Verification items for this drawing (mm, ordinates from the low corner). Coordinates: 2 decimals unless noted, no trailing zeros. Order: outer loops, then holes, each group sorted by start corner. A loop starts at its lowest first (then second) coordinate and runs counter-clockwise, first axis right, second up.
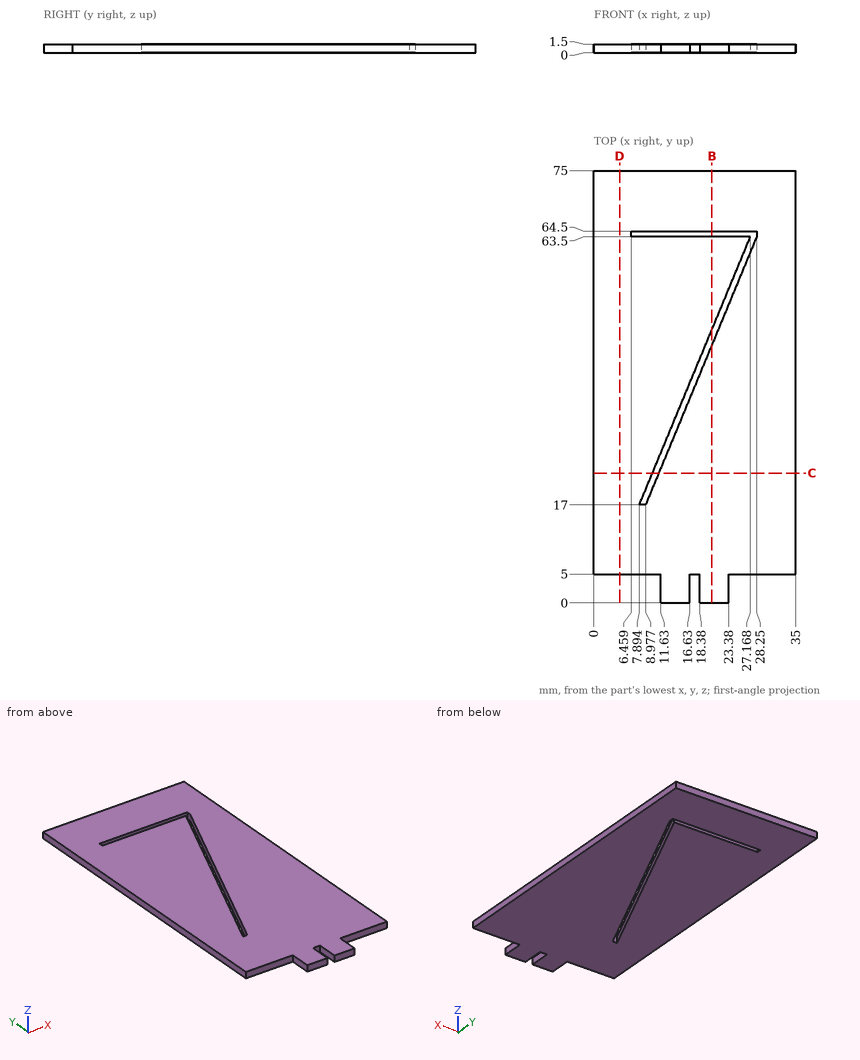
(1) Cross-section at B-B (x = 20.5). Enter the section's corners in (y, z), and give its area (3 significant figures).
Filled in:
outline: (0, 0) - (44.8, 0) - (44.8, 1.5) - (0, 1.5) - close; (47.41, 0) - (63.5, 0) - (63.5, 1.5) - (47.41, 1.5) - close; (64.5, 0) - (75, 0) - (75, 1.5) - (64.5, 1.5) - close
area: 107 mm2
(2) Cross-section at C-C (y = 22.5). Enter the section's corners in (x, z).
Filled in:
outline: (0, 0) - (10.17, 0) - (10.17, 1.5) - (0, 1.5) - close; (11.26, 0) - (35, 0) - (35, 1.5) - (11.26, 1.5) - close
(3) Cross-section at D-D (x = 4.5). Enter the section's corners in (y, z), and give its area (3 significant figures).
Filled in:
outline: (5, 0) - (75, 0) - (75, 1.5) - (5, 1.5) - close
area: 105 mm2
(4) Thickness scan on probe 1 along Y at (x, z) = (14.5, 1.05) (1 decimal); probe 2 along Y at (x, z) = (18, 0.95) (1 decimal); probe 3 along Y at (x, z) = (6.5, 0.45). Record the ranges inside material, lowest first.
Filled in:
probe 1: y = 0 to 30.3, 32.9 to 63.5, 64.5 to 75
probe 2: y = 5 to 38.8, 41.4 to 63.5, 64.5 to 75
probe 3: y = 5 to 63.5, 64.5 to 75
(5) Go/stop test with a flat-tipped pin: P1, Ø0.8, axis at y = 2, z = 0.5, coming from the -X side. Record where the tip stops, or that it passes through.
Filled in:
P1: stops at x = 11.63
